Can you work these out from the model? Positions are in its coordinate system, mm. Give positions to 0.01 mm unless a question says otherwise; leave off trailing zeros. Loops run counter-clockwise (first coordinate to the right, second up) from the corner with the lowest first, then second, coordinate; pieces in that order, holes last. Notation, with made-up numbers: (24.5, -29) - (58.5, -29) arc R25 ccw to (58.5, 10) - close; hole circle Ø11 at (36, 57.5). An arc over 180 degrees is marked (long way). Answer as a JSON object with one key per item and string values. Group by question number.
Item 1: Suppose I cut it at B-B on y = -4.5. Count the separate pieces of the cut face and the enclosed holes in it, and give its area (3 significant figures).
Item 2: Will these pins go through, and if not, where does the flat tip stop? pin 1 (0.9 mm diameter, centred on y = -9, z = 2, fed in from -X); pin 2 (5 mm diameter, centred on x = -6, y = 13, fed in from -Z); pin 3 (3.5 mm diameter, centred on y = -8, z = 1, fed in from -X); pin 4 (1.5 mm diameter, centred on y = 7, z = 1, fed in from -X).
Item 3: Suppose I cut it at C-C on z = -4. Write out the boundary of the cut face in (x, y).
Item 4: Suppose I cut it at A-A on x = 7. Write out the boundary of the cut face in (y, z), and give its area (3 significant figures).
Item 5: Please list where these lines run through material, in increasing order: L1, parallel to X at y = 13.4, z = -4; L2, parallel to Y at x = -12.5, z = 2; L3, parallel to X at y = -3, z = 0.5.
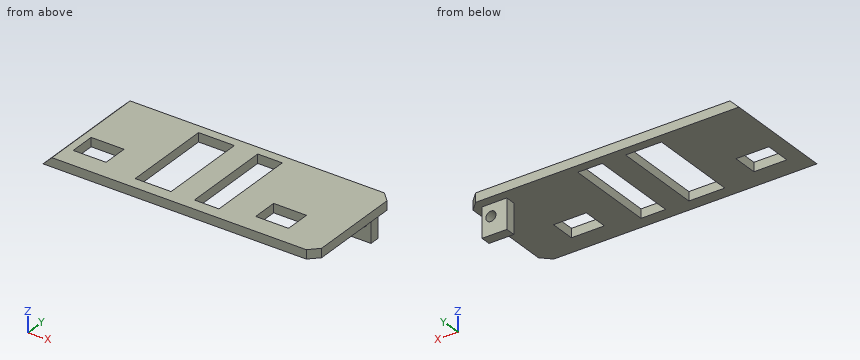
from build123d import *

# Parameters (mm, degrees)
SKETCH_1_W          = 91
SKETCH_1_H          = 37
EXTRUDE_1_DEPTH     = 3
CHAMFER_1_SIZE      = 3
SKETCH_2_W          = 11
SKETCH_2_H          = 8.5
CUT_EXTRUDE_1_DEPTH = 10
SKETCH_3_W          = 12
SKETCH_3_H          = 30
SKETCH_3_W_2        = 8.207535441
CUT_EXTRUDE_2_DEPTH = 10
SKETCH_4_W          = 8.305337468
SKETCH_4_H          = 3.319312894
EXTRUDE_2_DEPTH     = 10
SKETCH_5_R          = 1.683787266
CUT_EXTRUDE_3_DEPTH = 10
CHAMFER_2_SIZE      = 3
CHAMFER_3_SIZE      = 3


with BuildPart() as part:
    # 草图1 → 凸台-拉伸1 (new body)
    with BuildSketch(Plane.XY):
        Rectangle(SKETCH_1_W, SKETCH_1_H)
    extrude(amount=EXTRUDE_1_DEPTH)

    # 倒角1
    chamfer_1_edges = [part.edges().sort_by_distance(p)[0] for p in [
        (-45.5, 0, 3),
    ]]
    chamfer(chamfer_1_edges, length=CHAMFER_1_SIZE - 0.0001)  # a hair under: the kernel refuses the full size

    # 草图2 → 切除-拉伸1 (cut)
    with BuildSketch(Plane.XY.offset(3)):
        with Locations((-34.5, -7.75)):
            Rectangle(SKETCH_2_W, SKETCH_2_H)
        with Locations((26.5, -7.75)):
            Rectangle(SKETCH_2_W, SKETCH_2_H)
    extrude(amount=-CUT_EXTRUDE_1_DEPTH, mode=Mode.SUBTRACT)

    # 草图3 → 切除-拉伸2 (cut)
    with BuildSketch(Plane(origin=(0, 0, 0), x_dir=(-1, 0, 0), z_dir=(0, 0, -1))):
        with Locations((11.5, 0.5)):
            Rectangle(SKETCH_3_W, SKETCH_3_H)
        with Locations((-6.39623228, 0.5)):
            Rectangle(SKETCH_3_W_2, SKETCH_3_H)
    extrude(amount=-CUT_EXTRUDE_2_DEPTH, mode=Mode.SUBTRACT)

    # 草图4 → 凸台-拉伸2 (add)
    with BuildSketch(Plane(origin=(0, 0, 0), x_dir=(-1, 0, 0), z_dir=(0, 0, -1))):
        with Locations((-38.347331266, 13.840343553)):
            Rectangle(SKETCH_4_W, SKETCH_4_H)
    extrude(amount=EXTRUDE_2_DEPTH)

    # 草图5 → 切除-拉伸3 (cut)
    with BuildSketch(Plane(origin=(0, 15.5, 0), x_dir=(1, 0, 0), z_dir=(0, 1, 0))):
        with Locations(Location((39.5, 4, 0), (0, 0, 270))):
            Circle(SKETCH_5_R)
    extrude(amount=-CUT_EXTRUDE_3_DEPTH, mode=Mode.SUBTRACT)

    # 倒角2
    chamfer_2_edges = [part.edges().sort_by_distance(p)[0] for p in [
        (45.5, 18.5, 1.5),
    ]]
    chamfer(chamfer_2_edges, length=CHAMFER_2_SIZE)

    # 倒角3
    chamfer_3_edges = [part.edges().sort_by_distance(p)[0] for p in [
        (45.5, -18.5, 1.5),
    ]]
    chamfer(chamfer_3_edges, length=CHAMFER_3_SIZE)


solid = part.part
Worked out:
{
 "1": {"separate pieces": "5", "enclosed holes": "0", "area": "142 mm2"},
 "2": {"pin 1": "stops at x = -43.95", "pin 2": "stops at z = 0", "pin 3": "stops at x = -45.5", "pin 4": "stops at x = -45.25"},
 "3": {"outline": "(34.19, 12.18) - (37.82, 12.18) - (37.82, 15.5) - (34.19, 15.5) - close; (41.18, 12.18) - (42.5, 12.18) - (42.5, 15.5) - (41.18, 15.5) - close"},
 "4": {"outline": "(-18.5, 0) - (-14.5, 0) - (-14.5, 3) - (-18.5, 3) - close; (15.5, 0) - (18.5, 0) - (18.5, 3) - (15.5, 3) - close", "area": "21.0 mm2"},
 "5": {"L1": "x = 34.19 to 37.82, 41.18 to 42.5", "L2": "y = -18.5 to -14.5, 15.5 to 18.5", "L3": "x = -45 to -17.5, -5.5 to 2.29, 10.5 to 45.5"}
}
